Autodesk Inventor part; units mm, degrees
sketch "Sketch19" plane through (0, 0, 0) normal (0, 0, 1) x (1, 0, 0)
  circle A0 centre (0, 0) radius 12.5
  dimension "d130" = 25
extrude "Extrusion17" add sketch "Sketch19" along normal blind 50
sketch "Sketch20" plane through (0, 0, 50) normal (0, 0, 1) x (1, 0, 0)
  circle A0 centre (0, 0) radius 10
  dimension "d133" = 20
fillet "Fillet6" radius 10 1 edges at (-12.5, 0, 0)
extrude "Extrusion18" cut sketch "Sketch20" against normal blind 40
ref_plane "Work Plane3" through (10, 0, 0) normal (1, 0, 0) x (0, 1, 0)
sketch "Sketch21" plane through (10, 0, 0) normal (1, 0, 0) x (0, 1, 0)
  line L0 (0, 0) -> (0, 20)
  circle A0 centre (0, 20) radius 5
  dimension "d138" = 20
  dimension "d139" = 10
extrude "Extrusion19" add sketch "Sketch21" along normal blind 10
mirror "Mirror1" about plane through (0, 0, 0) normal (1, 0, 0) of "Extrusion19"
sketch "Sketch22" plane through (-20, 0, 20) normal (-1, 0, 0) x (0, 0, 1)
  circle A0 centre (0, 0) radius 2.5
  point P0 (-20, 0)
  dimension "d142" = 5
extrude "Extrusion20" cut sketch "Sketch22" against normal blind 3
properties part number "Waterkanon" material "S235"
Design review of the part built by this model. Coordinates are the model's own, in mm. A direction names the side the tool comes from. Give positions to 0.01 mm unless a question says otherwise; leave off trailing zeros. Order: outer loops, then holes, each group sorted by start corner. A loop starts at its lowest first (then second) coordinate and runs counter-clockwise, first axis right, second up. Notation, with made-up numbers: (56.5, 84) - (102.5, 84) arc R18 ccw to (102.5, 89) - close; hole circle Ø7 at (-25, -8). An arc over 180 degrees is marked (long way). Use a Markdown table: item, result. Add a question column.
(1) Add section A-A on z = 20. Give the boundary of the cut face in (x, y), then the cut area to 3 significant figures.
(2) Clearance check with flat-ended pins moving along their axes: P1, Ø1, axis at x = 4, y = -9.5, coming from the -Z side; P2, Ø1, axis at x = 8, y = 4, coming from the +Z side; P3, Ø3, axis at x = 12.5, z = 18, coming from the +Y side. State where each tip first meets the part, or that it passes through.
(3) Mouldability with a two-part tool opening along X and no side actions: class faces 1 (the face through (15.67, -1.08, 24.88)), 2 (the face through (-2.17, -9.76, 30.28)), 3 (the face through (0, 0, 10)), 4 (the face through (-17, 0, 20)) as +X half, -X half, draft (parallel to the pull), parting line (faces both ways), or undercut.
(4) Machinability: for faces 5 (the face through (-18.5, 0.1, 17.5)), 6 (the face through (-20, -2, 18)), which of the approach directions +Z, -Z, +X, -X, +Y, -Y give a long, thin tool a straight path to every point of the face, cutting with its end or side? Answer none if there is none.
(5) Wall thickness on probe 1 along Y at (x, z) = (0, 28); probe 2 along Y at (x, z) = (-19.25, 20); probe 3 along X at (y, z) = (7.5, 18): over which ranges is each line inside the solid? List them lowest first. Write a range as [from, to].
(6) Add section B-B on x = -14.5. Give the boundary of the cut face in (y, z), then the cut area to 3 significant figures.
(7) Add section C-C on z = 35.5. Give the boundary of the cut face in (x, y).
Report:
| question | item | result |
|---|---|---|
| 1 | outline | (-20, -5) - (-11.46, -5) arc R12.5 ccw to (11.46, -5) - (20, -5) - (20, 5) - (11.46, 5) arc R12.5 ccw to (-11.46, 5) - (-20, 5) - (-20, 2.5) - (-17, 2.5) - (-17, -2.5) - (-20, -2.5) - close; hole circle Ø20 at (0, 0) |
| 1 | area | 319 mm² |
| 2 | P1 | stops at z = 3.17 |
| 2 | P2 | stops at z = 10 |
| 2 | P3 | stops at y = 5.94 |
| 3 | face 1 | draft |
| 3 | face 2 | undercut |
| 3 | face 3 | undercut |
| 3 | face 4 | -X half |
| 4 | face 5 | -X |
| 4 | face 6 | +Z, -Z, -X, +Y, -Y |
| 5 | probe 1 | y = [-12.5, -10], [10, 12.5] |
| 5 | probe 2 | y = [-5, -2.5], [2.5, 5] |
| 5 | probe 3 | x = [-10, -6.61], [6.61, 10] |
| 6 | outline | circle Ø10 at (0, 20) |
| 6 | area | 78.5 mm² |
| 7 | outline | circle Ø25 at (0, 0); hole circle Ø20 at (0, 0) |
